Check sheet for the modelled part. Datum: model origin and axes. Units: mm. Round coordinates to 2 decimals unless told otherwise and drop trailing zeros. Write each loop counter-clockwise with the first axis right and the second up, starting at its lowest first coordinate (ties: lowest second). Pieces come first, ordered by that corner, then holes. Notation, with made-up numbers: (77, 1) -> (91, 1) arc R18 cw to (91, 27) -> close; hole circle Ø1 at (-11, -13). An arc over 180 degrees is marked (long way). Write item = value, one per line.
Autodesk Inventor part; units mm, degrees
ref_plane "YZ Plane" through (0, 0, 0) normal (1, 0, 0) x (0, 1, 0)
ref_plane "XZ Plane" through (0, 0, 0) normal (0, 1, 0) x (-1, 0, 0)
ref_plane "XY Plane" through (0, 0, 0) normal (0, 0, 1) x (1, 0, 0)
sketch "Boceto1" plane through (0, 0, 0) normal (0, 0, 1) x (1, 0, 0)
  line L0 (125, 125) -> (-125, 125)
  line L1 (-125, 125) -> (-125, -125)
  line L2 (-125, -125) -> (125, -125)
  line L3 (125, -125) -> (125, 125)
  line L4 (125, 125) -> (-125, -125) construction
  line L5 (-125, 125) -> (125, -125) construction
  point P0 (0, 0)
  dimension "d0" = 250
  dimension "d1" = 250
extrude "Extrusión1" add sketch "Boceto1" along normal blind 350
sketch "Boceto2" plane through (125, -125, 0) normal (1, 0, 0) x (0, 0, -1)
  line L0 (0, 0) -> (0, 250)
  line L1 (0, 250) -> (-350, 250)
  line L2 (-350, 0) -> (-350, 250)
  line L3 (0, 0) -> (-350, 0)
  line L4 (-325, 225) -> (-25, 225)
  line L5 (-25, 225) -> (-25, 25)
  line L6 (-25, 25) -> (-325, 25)
  line L7 (-325, 25) -> (-325, 225)
  line L8 (-30, 220) -> (-320, 220)
  line L9 (-320, 220) -> (-320, 30)
  line L10 (-320, 30) -> (-30, 30)
  line L11 (-30, 30) -> (-30, 220)
  point P0 (0, 125)
  dimension "d4" = 25
  dimension "d5" = 5
extrude "Extrusión2" cut sketch "Boceto2" against normal blind 5 contours L4 L5 L6 L7
sketch "Boceto3" plane through (125, -95, 30) normal (1, 0, 0) x (0, 0, -1)
  line L0 (-290, 0) -> (0, 0)
  line L1 (0, 0) -> (0, 190)
  line L2 (0, 190) -> (-290, 190)
  line L3 (-290, 190) -> (-290, 0)
  circle A0 centre (-263.8975, 95) radius 5
  point P0 (30, 95)
  dimension "d8" = 10
extrude "Extrusión3" add sketch "Boceto3" along normal blind 5 contours A0
fillet "Empalme1" radius 5 12 edges at (0, 125, 350) (0, 125, 0) (0, -125, 350) (0, -125, 0) (-125, 125, 175) (-125, 0, 0) (-125, 0, 350) (-125, -125, 175) (125, 0, 350) (125, 125, 175) (125, 0, 0) (125, -125, 175)
(1) Sectioned sample at A-A on z = 84. Enter the section's corners in (x, y), then the cut area to 3 significant figures.
Worked answers:
outline = (-125, -120) arc R5 ccw to (-120, -125) -> (120, -125) arc R5 ccw to (125, -120) -> (125, -100) -> (120, -100) -> (120, -95) -> (125, -95) -> (125, 95) -> (120, 95) -> (120, 100) -> (125, 100) -> (125, 120) arc R5 ccw to (120, 125) -> (-120, 125) arc R5 ccw to (-125, 120) -> close
area = 62,400 mm²
(2) Release check for a two-part mould opening along Z. For faces 1 (the cylindrical face through (127.465, -0.22, 298.893)), 2 (the flat face through (120, -96, 220)), 3 (the flat face through (-2, 2, 0)) record: pulls with the +Z half, pulls with the -Z half, needs draft (parallel to the pull), parting line crosses it, or undercut.
Worked answers:
face_1 = parting line crosses it
face_2 = undercut
face_3 = pulls with the -Z half
(3) Sectioned sample at B-B on y = -89. Enter the section's corners in (x, z), then the cut area to 3 significant figures.
Worked answers:
outline = (-125, 5) arc R5 ccw to (-120, 0) -> (120, 0) arc R5 ccw to (125, 5) -> (125, 25) -> (120, 25) -> (120, 30) -> (125, 30) -> (125, 320) -> (120, 320) -> (120, 325) -> (125, 325) -> (125, 345) arc R5 ccw to (120, 350) -> (-120, 350) arc R5 ccw to (-125, 345) -> close
area = 87,400 mm²
(4) Go/stop test with flat-tipped pins: P1, Ø1.5, axis at x = 121.5, y = -10.5, coming from the +Z side; P2, Ø1.5, axis at x = 122.5, z = 240, coming from the +Y side; P3, Ø2.5, axis at x = 123, y = -31.5, coming from the -Z side. Record where each tip stops, or that it passes through.
Worked answers:
P1 = 349.94
P2 = 124.68
P3 = 0.32
(5) Material ranges on L1, parallel to X at y = 34.5, z = 167, recorded low to high. Write a range as [from, to].
Worked answers:
L1 = [-125, 125]
(6) Sectioned sample at C-C on y = 0. Enter the section's corners in (x, z), then the cut area to 3 significant figures.
Worked answers:
outline = (-125, 5) arc R5 ccw to (-120, 0) -> (120, 0) arc R5 ccw to (125, 5) -> (125, 25) -> (120, 25) -> (120, 30) -> (125, 30) -> (125, 288.9) -> (130, 288.9) -> (130, 298.9) -> (125, 298.9) -> (125, 320) -> (120, 320) -> (120, 325) -> (125, 325) -> (125, 345) arc R5 ccw to (120, 350) -> (-120, 350) arc R5 ccw to (-125, 345) -> close
area = 87,500 mm²
